Build history of the part. All positions in model axes, mm. Face numbers are marked on the shaded views. Round coordinates to 2 decimals unless told otherwise and drop trailing zeros. Order: outer loops, then holes, each group sorted by start corner. A loop starts at its lowest first (then second) coordinate and runs counter-clockwise, first axis right, second up. Notation, with made-up numbers: (53.25, 12) -> (89.25, 12) arc R37 ccw to (89.25, 50) -> close; hole circle Ø5 at (28.25, 48). An arc over 180 degrees is marked (long way). Write item = value, one per line.
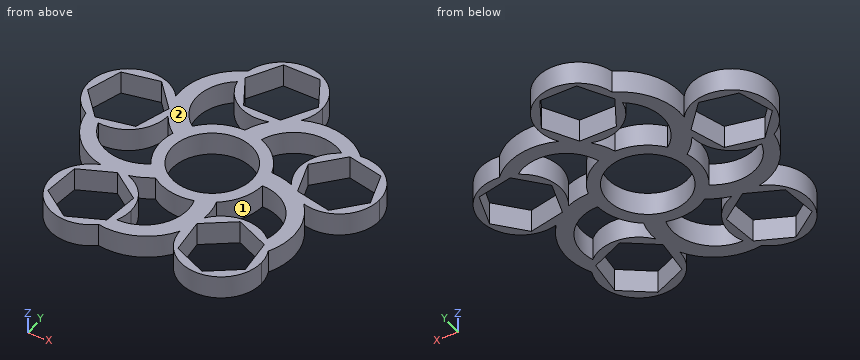
from build123d import *

# Parameters (mm, degrees)
F0_R     = 11.0236
F1_DEPTH = 6.35


with BuildPart() as f1:
    # F0 (on Top) → F1 (new body)
    with BuildSketch(Plane.XY):
        with BuildLine():
            ThreePointArc((-10.9013073569, 28.323810268), (-5.7416369548, 20.9657337998), (3.1731830809, 19.8301847253))
            ThreePointArc((3.1731830809, 19.8301847253), (5.9411817185, 22.3894795146), (9.2116796693, 24.2644860293))
            ThreePointArc((9.2116796693, 24.2644860293), (10.6266750815, 27.2301641638), (11.1125, 30.48))
            ThreePointArc((11.1125, 30.48), (1.2150273194, 41.5258754684), (-10.8468007628, 32.8954853473))
            ThreePointArc((-10.8468007628, 32.8954853473), (-11.1117102623, 30.6124813052), (-10.9013073569, 28.323810268))
        make_face()
        Polygon((10.0819790757, 30.48), (5.0409895379, 21.74875), (-5.0409895379, 21.74875), (-10.0819790757, 30.48), (-5.0409895379, 39.21125), (5.0409895379, 39.21125), align=None, mode=Mode.SUBTRACT)
        with BuildLine():
            ThreePointArc((-30.3062335558, -1.6152206797), (-21.7138611437, 1.0181468036), (-17.8790589041, 9.1457405282))
            ThreePointArc((-17.8790589041, 9.1457405282), (-19.4577342712, 12.5691292531), (-20.2303319881, 16.2589665183))
            ThreePointArc((-20.2303319881, 16.2589665183), (-37.3389530107, 16.7504560982), (-34.6373114666, -0.1506565358))
            ThreePointArc((-34.6373114666, -0.1506565358), (-32.5479071329, -1.1080874889), (-30.3062335558, -1.6152206797))
        make_face()
        Polygon((-22.2420418444, 1.9264674079), (-32.103705488, -0.1696939086), (-38.8498662602, 7.3226766721), (-35.7343633889, 16.9112085692), (-25.8726997453, 19.0073698857), (-19.1265389731, 11.514999305), align=None, mode=Mode.SUBTRACT)
        with BuildLine():
            ThreePointArc((-14.2230491705, -14.1778062266), (-11.1849106676, -13.1482774657), (-8.3989318902, -11.5581399608))
            ThreePointArc((-8.3989318902, -11.5581399608), (-10.3627655441, -9.835941568), (-11.980250366, -7.7850020821))
            ThreePointArc((-11.980250366, -7.7850020821), (-22.7179291909, -9.3773746133), (-30.3062335558, -1.6152206797))
            ThreePointArc((-30.3062335558, -1.6152206797), (-32.5479071329, -1.1080874889), (-34.6373114666, -0.1506565358))
            ThreePointArc((-34.6373114666, -0.1506565358), (-30.3789037171, -9.207206787), (-21.7147124417, -14.215892099))
            ThreePointArc((-21.7147124417, -14.215892099), (-17.9721871235, -13.5464815853), (-14.2230491705, -14.1778062266))
        make_face()
        with BuildLine():
            ThreePointArc((-13.5878570147, 4.4161972328), (-12.556806984, 6.8161025973), (-11.1060779195, 8.9881972328))
            ThreePointArc((-11.1060779195, 8.9881972328), (-15.9386394287, 18.7082664756), (-10.9013073569, 28.323810268))
            ThreePointArc((-10.9013073569, 28.323810268), (-11.1117102623, 30.6124813052), (-10.8468007628, 32.8954853473))
            ThreePointArc((-10.8468007628, 32.8954853473), (-18.1441715308, 26.0468709702), (-20.2303319881, 16.2589665183))
            ThreePointArc((-20.2303319881, 16.2589665183), (-18.4808363051, 13.0358684619), (-17.8757026167, 9.4188379885))
            ThreePointArc((-17.8757026167, 9.4188379885), (-17.8765417202, 9.2822789468), (-17.8790589041, 9.1457405282))
            ThreePointArc((-17.8790589041, 9.1457405282), (-15.9610824387, 6.5744409909), (-13.5878570147, 4.4161972328))
        make_face()
        with BuildLine():
            ThreePointArc((-20.2303319881, 16.2589665183), (-19.4577342712, 12.5691292531), (-17.8790589041, 9.1457405282))
            ThreePointArc((-17.8790589041, 9.1457405282), (-17.8765417202, 9.2822789468), (-17.8757026167, 9.4188379885))
            ThreePointArc((-17.8757026167, 9.4188379885), (-18.4808363051, 13.0358684619), (-20.2303319881, 16.2589665183))
        make_face()
        with BuildLine():
            ThreePointArc((0.0011744209, 14.2874999517), (2.6022320378, 14.0485246439), (5.1163167301, 13.3400134695))
            ThreePointArc((5.1163167301, 13.3400134695), (12.8673082895, 20.9397191658), (23.5688550875, 19.1202981162))
            ThreePointArc((23.5688550875, 19.1202981162), (25.6804925176, 20.0276414155), (27.933619926, 20.4811845569))
            ThreePointArc((27.933619926, 20.4811845569), (19.1651890134, 25.3050583472), (9.2116796693, 24.2644860293))
            ThreePointArc((9.2116796693, 24.2644860293), (6.5773827127, 21.5231203591), (3.1731830809, 19.8301847253))
            ThreePointArc((3.1731830809, 19.8301847253), (1.3204192232, 17.2115054551), (0.0011744209, 14.2874999517))
        make_face()
        with BuildLine():
            ThreePointArc((25.9234631172, -1.2626894327), (23.1295865065, 1.2683300774), (19.8401939006, 3.1099876352))
            ThreePointArc((19.8401939006, 3.1099876352), (22.5022269053, 0.3955472739), (25.9234631172, -1.2626894327))
        make_face()
        with BuildLine():
            ThreePointArc((13.5885828467, 4.4139633516), (14.1116890143, 2.2344774365), (14.2875, 0))
            ThreePointArc((14.2875, 0), (14.2826580685, -0.3719337948), (14.2681355559, -0.7436154983))
            ThreePointArc((14.2681355559, -0.7436154983), (23.8910732953, -5.7668083163), (25.4676608769, -16.5068161571))
            ThreePointArc((25.4676608769, -16.5068161571), (26.9831274861, -18.234718196), (28.1107273058, -20.2374171613))
            ThreePointArc((28.1107273058, -20.2374171613), (29.9889097419, -10.4074848243), (25.9234631172, -1.2626894327))
            ThreePointArc((25.9234631172, -1.2626894327), (22.5022269053, 0.3955472739), (19.8401939006, 3.1099876352))
            ThreePointArc((19.8401939006, 3.1099876352), (16.777146398, 4.0628543779), (13.5885828467, 4.4139633516))
        make_face()
        with BuildLine():
            ThreePointArc((23.5688550875, 19.1202981162), (18.1653343546, 11.9393892838), (19.8401939006, 3.1099876352))
            ThreePointArc((19.8401939006, 3.1099876352), (23.1295865065, 1.2683300774), (25.9234631172, -1.2626894327))
            ThreePointArc((25.9234631172, -1.2626894327), (35.6751577744, 0.5434626743), (40.1007026167, 9.4188379885))
            ThreePointArc((40.1007026167, 9.4188379885), (36.4637830657, 17.6409638207), (27.933619926, 20.4811845569))
            ThreePointArc((27.933619926, 20.4811845569), (25.6804925176, 20.0276414155), (23.5688550875, 19.1202981162))
        make_face()
        Polygon((19.1265389731, 11.514999305), (25.8726997453, 19.0073698857), (35.7343633889, 16.9112085692), (38.8498662602, 7.3226766721), (32.103705488, -0.1696939086), (22.2420418444, 1.9264674079), align=None, mode=Mode.SUBTRACT)
        with BuildLine():
            ThreePointArc((9.0887310931, -17.9081066622), (9.048427485, -14.7005233582), (8.3970316373, -11.5595205754))
            ThreePointArc((8.3970316373, -11.5595205754), (6.1522656603, -12.8950487977), (3.7018759995, -13.799593122))
            ThreePointArc((3.7018759995, -13.799593122), (1.8981870347, -24.5038027118), (-7.8289750516, -29.3220715473))
            ThreePointArc((-7.8289750516, -29.3220715473), (-9.0040026085, -31.2973170358), (-10.5602350025, -32.9885962071))
            ThreePointArc((-10.5602350025, -32.9885962071), (-0.6310235074, -31.737237706), (6.8099016433, -25.0448710159))
            ThreePointArc((6.8099016433, -25.0448710159), (7.3297583374, -21.2786586997), (9.0887310931, -17.9081066622))
        make_face()
        with BuildLine():
            ThreePointArc((-21.7147124417, -14.215892099), (-17.9667228421, -14.6213304272), (-14.2230491705, -14.1778062266))
            ThreePointArc((-14.2230491705, -14.1778062266), (-17.9721871235, -13.5464815853), (-21.7147124417, -14.215892099))
        make_face()
        with BuildLine():
            ThreePointArc((-10.5602350025, -32.9885962071), (-9.0040026085, -31.2973170358), (-7.8289750516, -29.3220715473))
            ThreePointArc((-7.8289750516, -29.3220715473), (-7.0626689668, -27.0461991355), (-6.8031944899, -24.6588379885))
            ThreePointArc((-6.8031944899, -24.6588379885), (-8.8459045981, -18.2380461706), (-14.2230491705, -14.1778062266))
            ThreePointArc((-14.2230491705, -14.1778062266), (-17.9667228421, -14.6213304272), (-21.7147124417, -14.215892099))
            ThreePointArc((-21.7147124417, -14.215892099), (-27.4690014556, -30.3352789746), (-10.5602350025, -32.9885962071))
        make_face()
        Polygon((-8.7053483012, -20.5581276637), (-9.7592020807, -30.5848766032), (-18.9695482694, -34.685586928), (-27.1260406785, -28.7595483134), (-26.0721868991, -18.7327993739), (-16.8618407104, -14.6320890491), align=None, mode=Mode.SUBTRACT)
        with BuildLine():
            ThreePointArc((6.8099016433, -25.0448710159), (8.3536888883, -21.6056084179), (9.0887310931, -17.9081066622))
            ThreePointArc((9.0887310931, -17.9081066622), (7.3297583374, -21.2786586997), (6.8099016433, -25.0448710159))
        make_face()
        with BuildLine():
            ThreePointArc((28.1107273058, -20.2374171613), (26.9831274861, -18.234718196), (25.4676608769, -16.5068161571))
            ThreePointArc((25.4676608769, -16.5068161571), (16.968431003, -13.5867854175), (9.0887310931, -17.9081066622))
            ThreePointArc((9.0887310931, -17.9081066622), (8.3536888883, -21.6056084179), (6.8099016433, -25.0448710159))
            ThreePointArc((6.8099016433, -25.0448710159), (18.1087401348, -35.7696610737), (29.0281944899, -24.6588379885))
            ThreePointArc((29.0281944899, -24.6588379885), (28.7964104226, -22.4010344007), (28.1107273058, -20.2374171613))
        make_face()
        Polygon((16.8618407104, -14.6320890491), (26.0721868991, -18.7327993739), (27.1260406785, -28.7595483134), (18.9695482694, -34.685586928), (9.7592020807, -30.5848766032), (8.7053483012, -20.5581276637), align=None, mode=Mode.SUBTRACT)
        with BuildLine():
            ThreePointArc((14.2681355559, -0.7436154983), (14.2826580685, -0.3719337948), (14.2875, 0))
            ThreePointArc((14.2875, 0), (14.1116890143, 2.2344774365), (13.5885828467, 4.4139633516))
            ThreePointArc((13.5885828467, 4.4139633516), (10.3627655441, 9.835941568), (5.1163167301, 13.3400134695))
            ThreePointArc((5.1163167301, 13.3400134695), (2.6022320378, 14.0485246439), (0.0011744209, 14.2874999517))
            ThreePointArc((0.0011744209, 14.2874999517), (-6.1522656603, 12.8950487977), (-11.1060779195, 8.9881972328))
            ThreePointArc((-11.1060779195, 8.9881972328), (-12.556806984, 6.8161025973), (-13.5878570147, 4.4161972328))
            ThreePointArc((-13.5878570147, 4.4161972328), (-14.1650748299, -1.8663631244), (-11.980250366, -7.7850020821))
            ThreePointArc((-11.980250366, -7.7850020821), (-10.3627655441, -9.835941568), (-8.3989318902, -11.5581399608))
            ThreePointArc((-8.3989318902, -11.5581399608), (-2.6022320378, -14.0485246439), (3.7018759995, -13.799593122))
            ThreePointArc((3.7018759995, -13.799593122), (6.1522656603, -12.8950487977), (8.3970316373, -11.5595205754))
            ThreePointArc((8.3970316373, -11.5595205754), (12.556806984, -6.8161025973), (14.2681355559, -0.7436154983))
        make_face()
        Circle(F0_R, mode=Mode.SUBTRACT)
        with BuildLine():
            ThreePointArc((9.2116796693, 24.2644860293), (5.9411817185, 22.3894795146), (3.1731830809, 19.8301847253))
            ThreePointArc((3.1731830809, 19.8301847253), (6.5773827127, 21.5231203591), (9.2116796693, 24.2644860293))
        make_face()
    extrude(amount=F1_DEPTH)


solid = f1.part
Q1. Cut at C-C, the plane z = 5. Give the number of separate pieces and of enclosed holes in the cut face, and give its area (3 significant figures).
Check values:
separate_pieces = 1
enclosed_holes = 11
area = 1,470 mm²
Q2. Cut at A-A, the plane y = 34. List the corners of the cut face in (x, z), and give its area (3 significant figures).
Check values:
outline = (-10.54, 0) -> (-8.05, 0) -> (-8.05, 6.35) -> (-10.54, 6.35) -> close; (8.05, 0) -> (10.54, 0) -> (10.54, 6.35) -> (8.05, 6.35) -> close
area = 31.6 mm²
Q3. Mould opens along Y. For the marked faces 1 and 2 say: released by +Y, released by -Y, zero draft, split by the parting line, or undercut.
Check values:
face_1 = undercut
face_2 = zero draft
Q4. Cut at B-B, the plane y = -4. List the corners of the cut face in (x, z), and give its area (3 significant figures).
Check values:
outline = (-33.63, 0) -> (-29.27, 0) -> (-29.27, 6.35) -> (-33.63, 6.35) -> close; (-13.72, 0) -> (-10.27, 0) -> (-10.27, 6.35) -> (-13.72, 6.35) -> close; (10.27, 0) -> (13.72, 0) -> (13.72, 6.35) -> (10.27, 6.35) -> close; (22.35, 0) -> (27.88, 0) -> (27.88, 6.35) -> (22.35, 6.35) -> close
area = 107 mm²
Q5. Probe probe 1 along Y at (x, z) = (19, 2); probe 2 along X at (y, z) = (-32, 5.75); probe 3 along X at (y, z) = (-19, 1). List the from-to ranges inside material, lowest first.
Check values:
probe_1 = -35.72 to -34.66, -15.58 to -13.6, -1.77 to 3.44, 4.55 to 14.29, 21.21 to 25.34
probe_2 = -26.26 to -22.67, -12.94 to -1.24, 9.57 to 12.94, 22.67 to 26.26
probe_3 = -27.48 to -26.1, -10.85 to -8.35, 4.14 to 10.85, 26.1 to 28.71
Q6. Flat gauge pins, fed straight in: pin 1 (1.5 mm diameter, centred on x = -2, z = 4, fed in from -Y); pin 2 (1 mm diameter, centred on x = -2.5, z = 5.5, fed in from +Y); pin 3 (1 mm diameter, centred on y = -28, z = 1.5, fed in from +X). Where does each tip first touch, or does it go through?
Check values:
pin_1 = -32.54
pin_2 = 41.41
pin_3 = 28.66
